from build123d import *

# Parameters (mm, degrees)
SKETCH2_R           = 17.4625
BOSS_EXTRUDE1_DEPTH = 18
SKETCH13_R          = 0.8
CUT_EXTRUDE6_DEPTH  = 10
SKETCH16_R          = 11
CUT_EXTRUDE9_DEPTH  = 15
CUT_EXTRUDE11_DEPTH = 22
SKETCH21_W          = 16.25
SKETCH21_H          = 2.78436417
CUT_EXTRUDE12_DEPTH = 31.559414466
CUT_EXTRUDE13_REACH = 32.559
SKETCH24_W          = 16.25
SKETCH24_H          = 6.70136321


with BuildPart() as part:
    # Sketch2 → Boss-Extrude1 (new body)
    with BuildSketch(Plane.XY):
        Circle(SKETCH2_R)
    extrude(amount=BOSS_EXTRUDE1_DEPTH)

    # Sketch13 → Cut-Extrude6 (cut)
    with BuildSketch(Plane.XY.offset(18)):
        with Locations((0, 13.5)):
            Circle(SKETCH13_R)
        with Locations((11.691342951, -6.75)):
            Circle(SKETCH13_R)
        with Locations((-11.691342951, -6.75)):
            Circle(SKETCH13_R)
    extrude(amount=-CUT_EXTRUDE6_DEPTH, mode=Mode.SUBTRACT)

    # Sketch16 → Cut-Extrude9 (cut)
    with BuildSketch(Plane.XY.offset(18)):
        Circle(SKETCH16_R)
    extrude(amount=-CUT_EXTRUDE9_DEPTH, mode=Mode.SUBTRACT)

    # Sketch20 → Cut-Extrude11 (cut)
    with BuildSketch(Plane(origin=(5.95728493, 0, -11.08430825), x_dir=(0, 0, 1), z_dir=(0, 1, 0))):
        Polygon((16.52930825, -11.021800725), (16.52930825, -6.906800725), (14.92930825, -6.906800725), (14.92930825, -4.926800725), (16.52930825, -4.926800725), (16.52930825, -0.811800725), (18.05430825, -0.811800725), (18.05430825, 1.028199275), (22.11430825, 1.028199275), (22.11430825, -0.811800725), (23.63930825, -0.811800725), (23.63930825, -11.021800725), (22.11430825, -11.021800725), (22.11430825, -12.861800725), (18.05430825, -12.861800725), (18.05430825, -11.021800725), align=None)
    extrude(amount=-CUT_EXTRUDE11_DEPTH, mode=Mode.SUBTRACT)

    # Sketch21 → Cut-Extrude12 (cut, through all)
    with BuildSketch(Plane.XY.offset(18)):
        with Locations((0, -16.852182085)):
            Rectangle(SKETCH21_W, SKETCH21_H)
    extrude(amount=-CUT_EXTRUDE12_DEPTH, mode=Mode.SUBTRACT)

    # Cut-Extrude13: up to this face of the body (flat: up to its plane)
    cut_extrude13_end = Plane(part.part.faces().sort_by_distance((0, 0, 3))[0])
    # Sketch24 → Cut-Extrude13 (cut, up to the picked face)
    with BuildSketch(Plane.XY.offset(18), mode=Mode.PRIVATE) as cut_extrude13_sk1:
        with Locations((0.005436819, -10.109318395)):
            Rectangle(SKETCH24_W, SKETCH24_H)
    cut_extrude13_tool1 = split(extrude(cut_extrude13_sk1.sketch, amount=-CUT_EXTRUDE13_REACH, mode=Mode.PRIVATE), bisect_by=cut_extrude13_end, keep=Keep.BOTH, mode=Mode.PRIVATE)
    add(cut_extrude13_tool1.solids().sort_by(Axis((0.005437, -10.109318, 18), (0, 0, -1)))[0], mode=Mode.SUBTRACT)


solid = part.part
Can you work these out from the model? Positions are in its coordinate system, mm. A direction names the side the tool comes from. Give positions to 0.01 mm unless a question says otherwise; leave off trailing zeros. Write each loop counter-clockwise with the first axis right and the second up, starting at its lowest first coordinate (ties: lowest second). Pieces come first, ordered by that corner, then holes. Notation, with made-up numbers: M 55.5,-40 L 75.5,-40 A24 ccw 75.5,-29 Z; hole C -37.5,75.25 d2. An arc over 180 degrees is marked long. Answer in a Markdown table with one row per item. Add a question column.
Item 1: Please list where these lines run through material, in increasing order: L1, parallel to Y at x = 0, z = 14.5; L2, parallel to Y at x = 0, z = 9; L3, parallel to Z at x = 5.5, y = -6.5.
Item 2: Imagine slicing it at B-B, the plane x = 0. Write out the boundary of the cut face in (y, z) (1 decimal).
Item 3: For pin 1 Ø1.8 at (y, z) = (-14.5, 5) entering from -X; pin 2 Ø1.8 at (y, z) = (-14, 4.5) entering from +X; pin 3 Ø10 at (y, z) = (-5.5, 3.5) entering from -X, each with a flat end and sliding along its axis, tell me the tip position at first contact or that it passes through.
Item 4: We'd pull the mould along X, two halves only. Please class faces 1 (the flat face through (0, -15.46, 13)), 2 (the flat face through (-6, -14, 6.97)), 3 (the cylindrical face through (0.65, 17.45, 8.87)), 4 (the flat face through (0, -13.46, 14)): released by +X, released by -X, zero draft, split by the parting line, or undercut.
Item 5: Imagine slicing it at A-A, the plane z = 16. State how many separate pieces and enclosed holes the cut face has, plus the area to 3 significant figures.
Item 6: Imagine slicing it at D-D, the plane y = 13.5. Write out the boundary of the cut face in (x, z).
Item 7: On a 3-axis mill with a long thin cutter (end or side, diameter ignored), from which of +Z, -Z, +X, -X, +Y, -Y can I reach the whole of each face in a straight line? I mean faces 5 (the flat face through (0, 1, 0)), 6 (the flat face through (0, -14, 12.555)), 7 (the flat face through (-8.12, -10, 11)). Say none if no direction works.
Evaluation:
| question | item | result |
|---|---|---|
| 1 | L1 | y = -15.46 to -13.46, 11 to 12.7, 14.3 to 17.46 |
| 1 | L2 | y = 11 to 12.7, 14.3 to 17.46 |
| 1 | L3 | z = 0 to 3 |
| 2 | outline | M -15.5,0 L 17.5,0 L 17.5,18 L 14.3,18 L 14.3,8 L 12.7,8 L 12.7,18 L 11,18 L 11,3 L -13.5,3 L -13.5,3.8 L -15.5,3.8 Z; M -15.5,12.6 L -13.5,12.6 L -13.5,18 L -15.5,18 Z |
| 3 | pin 1 | stops at x = -10.95 |
| 3 | pin 2 | stops at x = 11.55 |
| 3 | pin 3 | stops at x = -17.46 |
| 4 | face 1 | zero draft |
| 4 | face 2 | undercut |
| 4 | face 3 | split by the parting line |
| 4 | face 4 | undercut |
| 5 | separate pieces | 1 |
| 5 | enclosed holes | 4 |
| 5 | area | 492 mm² |
| 6 | outline | M -11.08,0 L 11.08,0 L 11.08,18 L 0.8,18 L 0.8,8 L -0.8,8 L -0.8,18 L -11.08,18 Z |
| 7 | face 5 | -Z, +X, -X, +Y, -Y |
| 7 | face 6 | -Y |
| 7 | face 7 | +Z |
